Could you check a few things on this model? Use its own coordinates, in mm. Face numbers are marked on the shaded views. Coordinates: 2 decimals unless noted, no trailing zeros. Write each loop counter-clockwise with the first axis right and the second up, starting at its lowest first coordinate (ties: lowest second). Pieces come first, ordered by that corner, then holes.
Item 1: For P1, Ø5, axis at y = 4.5, z = 8, coming from the +X side; P2, Ø2, axis at x = -0.5, z = 23.5, coming from the +Y side; P3, Ø4, axis at y = -7, z = 11, coming from the +X side, each with a flat end and sliding along its axis, tell me the tip position at first contact or that it passes through.
Item 2: I want a section at A-A on x = 0. Please give me the cut outline in (y, z).
Item 3: Thinking about a two-plate mould opening in Y: for the marked faces 1 and 2, which applies, +Y half, -Y half, draft (parallel to the pull), parting line (faces both ways), or undercut?
Item 4: If I drill on probe 1 along Y at (x, z) = (0, 14); probe 2 along Y at (x, z) = (5, 25); probe 3 along Y at (x, z) = (8.25, 6), over which ranges is the centre line in solid material (lowest first)?
Item 5: I want a section at B-B on y = 0. Please give me the cut outline in (x, z), then the cut area to 3 significant figures.
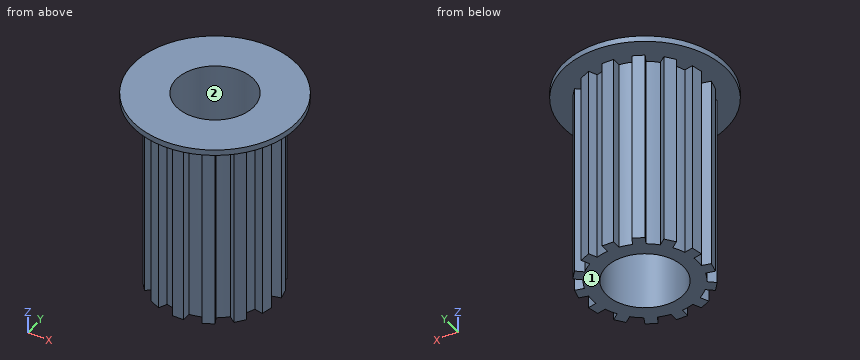
from build123d import *

# Parameters (mm, degrees)
F0_R            = 9.25
F0_R_2          = 6.75
F1_DEPTH        = 35
F2_W            = 2
F2_H            = 3
F3_DEPTH        = 35
F3_COPIES_COUNT = 14
F4_R            = 14.25
F4_R_2          = 6.75
F5_DEPTH        = 1


# Not quite as in the source:
# - a pattern or mirror of a feature is missing from the dataset's text; its kind, count and spacing are read off the source's solid


with BuildPart() as f1:
    # F0 (on Top) → F1 (new body)
    with BuildSketch(Plane.XY):
        Circle(F0_R)
        Circle(F0_R_2, mode=Mode.SUBTRACT)
    extrude(amount=F1_DEPTH)

    # F2 (on face) → F3 (join)
    with BuildSketch(Plane.XY.offset(35)):
        with Locations((0, 9.25)):
            Rectangle(F2_W, F2_H)
    f3 = extrude(amount=-F3_DEPTH)

    # F3_copies: F3 ×14 about axis
    f3_copies_axis = Axis((0, 0, 0), (0, 0, 1))
    for i in range(1, F3_COPIES_COUNT):
        add(f3.rotate(f3_copies_axis, i * 360 / F3_COPIES_COUNT))

    # F4 (on face) → F5 (join)
    with BuildSketch(Plane.XY.offset(35)):
        Circle(F4_R)
        Circle(F4_R_2, mode=Mode.SUBTRACT)
    extrude(amount=-F5_DEPTH)


solid = f1.part
Response values:
1. P1: stops at x = 10.57
1. P2: stops at y = 10.75
1. P3: stops at x = 9.03
2. outline: (-14.25, 34) - (-10.75, 34) - (-10.75, 0) - (-6.75, 0) - (-6.75, 35) - (-14.25, 35) - close; (6.75, 0) - (10.75, 0) - (10.75, 34) - (14.25, 34) - (14.25, 35) - (6.75, 35) - close
3. face 1: draft
3. face 2: undercut
4. probe 1: y = -10.75 to -6.75, 6.75 to 10.75
4. probe 2: y = -9.52 to -8.08, -7.78 to -4.53, 4.53 to 7.78, 8.08 to 9.52
4. probe 3: y = -6.9 to -5.3, -4.18 to 4.18, 5.3 to 6.9
5. outline: (-14.25, 34) - (-9.25, 34) - (-9.25, 0) - (-6.75, 0) - (-6.75, 35) - (-14.25, 35) - close; (6.75, 0) - (9.25, 0) - (9.25, 34) - (14.25, 34) - (14.25, 35) - (6.75, 35) - close
5. area: 185 mm2
